```python
from build123d import *

# Parameters (mm, degrees)
SKETCH1_W           = 50.8
SKETCH1_H           = 25.4
BOSS_EXTRUDE1_DEPTH = 609.6
SKETCH2_W           = 44.45
SKETCH2_H           = 19.05
CUT_EXTRUDE1_DEPTH  = 609.6
SKETCH6_R           = 14.2875
CUT_EXTRUDE5_DEPTH  = 25.4
CUT_EXTRUDE6_DEPTH  = 25.4
SKETCH8_R           = 14.2875
CUT_EXTRUDE7_DEPTH  = 3.175


with BuildPart() as part:
    # Sketch1 → Boss-Extrude1 (new body)
    with BuildSketch(Plane.XY):
        with Locations((25.4, 12.7)):
            Rectangle(SKETCH1_W, SKETCH1_H)
    extrude(amount=BOSS_EXTRUDE1_DEPTH)

    # Sketch2 → Cut-Extrude1 (cut)
    with BuildSketch(Plane(origin=(0, 0, 0), x_dir=(-1, 0, 0), z_dir=(0, 0, -1))):
        with Locations((-25.4, 12.7)):
            Rectangle(SKETCH2_W, SKETCH2_H)
    extrude(amount=-CUT_EXTRUDE1_DEPTH, mode=Mode.SUBTRACT)

    # Sketch6 → Cut-Extrude5 (cut)
    with BuildSketch(Plane(origin=(0, 25.4, 0), x_dir=(1, 0, 0), z_dir=(0, 1, 0))):
        with Locations((25.4, -25.4)):
            Circle(SKETCH6_R)
    extrude(amount=-CUT_EXTRUDE5_DEPTH, mode=Mode.SUBTRACT)

    # Sketch7 → Cut-Extrude6 (cut)
    with BuildSketch(Plane(origin=(0, 25.4, 0), x_dir=(1, 0, 0), z_dir=(0, 1, 0))):
        Polygon((50.8, -566.973738736), (50.8, -609.6), (0, -609.6), align=None)
    extrude(amount=-CUT_EXTRUDE6_DEPTH, mode=Mode.SUBTRACT)

    # Sketch8 → Cut-Extrude7 (cut)
    with BuildSketch(Plane.XZ):
        with Locations((25.4, 522.762581257)):
            Circle(SKETCH8_R)
    extrude(amount=-CUT_EXTRUDE7_DEPTH, mode=Mode.SUBTRACT)


solid = part.part
```
Geometry: final body of the model. Coordinates: model frame, mm. A direction names the side the tool comes from. Coordinates: 2 decimals unless noted, no trailing zeros. Order: outer loops, then holes, each group sorted by start corner. A loop starts at its lowest first (then second) coordinate and runs counter-clockwise, first axis right, second up. Notation, with made-up numbers: (50, 50.25) - (96, 50.25) arc R27 ccw to (96, 86.25) - close; hole circle Ø4 at (33.5, -19.5). An arc over 180 degrees is marked (long way). Return JSON: item names as keys, results as strings. Group by question number.
1. Cut plane A-A (y = 10.5). Output: boundary loops of the cut face in (x, z) (3 decimals).
2. Set-up query: faces 1 (the face through (23.54, 1.57, 536.93)), 2 (the face through (26, 3.175, 299)), 3 (the face through (0, 13, 301)). Return all of +Z, -Z, +X, -X, +Y, -Y with unobstructed straight access to the full face (end or side cutting, diameter ignored); none if empty.
3. Cut plane C-C (z = 316.5). Output: boundary loops of the cut face in (x, y) (3 decimals).
4. Cut plane B-B (z = 25.4). Output: boundary loops of the cut face in (x, y) (1 decimal), plus the area to 3 significant figures.
5. Cut plane D-D (x = 25.4). Output: boundary loops of the cut face in (y, z) (1 decimal).
6. Material intervals for line 1 along X through (y, z) = (23.9, 25.4); line 2 along Y through (x, z) = (31, 156.5) (3 decimals); line 3 along X through (y, z) = (6, 221.5) (3 decimals), sorted ascending. Write a range as [from, to].
7. Pin query (flat end, axial travel): pin 1 (5.5 mm diameter, centred on y = 8.5, z = 170.5, fed in from -X); pin 2 (17 mm diameter, centred on x = 25.4, z = 522.76, fed in from -Y) (3 decimals); pin 3 (5 mm diameter, centred on x = 17.5, y = 22, fed in from +Z) (3 decimals). Return the tip coordinate at first contact, or that it passes through.
8. Pull-direction query (Z, two-part tool) for faces 4 (the face through (14.87, 1.61, 15.744)), 5 (the face through (47.625, 13, 281)), 6 (the face through (25, 23, 0)); classes: pulls with the +Z half, pulls with the -Z half, needs draft (parallel to the pull), parting line crosses it, or undercut.
Resolved:
{
 "1": {"outline": "(0, 0) - (3.175, 0) - (3.175, 606.936) - (0, 609.6) - close; (47.625, 0) - (50.8, 0) - (50.8, 566.974) - (47.625, 569.638) - close"},
 "2": {"face 1": "-Y", "face 2": "+Z, -Z", "face 3": "+Z, -Z, -X, +Y, -Y"},
 "3": {"outline": "(0, 0) - (50.8, 0) - (50.8, 25.4) - (0, 25.4) - close; hole (3.175, 3.175) - (47.625, 3.175) - (47.625, 22.225) - (3.175, 22.225) - close"},
 "4": {"outline": "(0, 0) - (11.1, 0) - (11.1, 3.2) - (3.2, 3.2) - (3.2, 22.2) - (11.1, 22.2) - (11.1, 25.4) - (0, 25.4) - close; (39.7, 0) - (50.8, 0) - (50.8, 25.4) - (39.7, 25.4) - (39.7, 22.2) - (47.6, 22.2) - (47.6, 3.2) - (39.7, 3.2) - close", "area": "262 mm²"},
 "5": {"outline": "(0, 0) - (3.2, 0) - (3.2, 11.1) - (0, 11.1) - close; (0, 39.7) - (3.2, 39.7) - (3.2, 508.5) - (0, 508.5) - close; (0, 537.1) - (3.2, 537.1) - (3.2, 588.3) - (0, 588.3) - close; (22.2, 0) - (25.4, 0) - (25.4, 11.1) - (22.2, 11.1) - close; (22.2, 39.7) - (25.4, 39.7) - (25.4, 588.3) - (22.2, 588.3) - close"},
 "6": {"line 1": "x = [0, 11.11], [39.69, 50.8]", "line 2": "y = [0, 3.175], [22.225, 25.4]", "line 3": "x = [0, 3.175], [47.625, 50.8]"},
 "7": {"pin 1": "stops at x = 0", "pin 2": "stops at y = 22.225", "pin 3": "stops at z = 597.005"},
 "8": {"face 4": "undercut", "face 5": "needs draft", "face 6": "pulls with the -Z half"}
}
